```python
from build123d import *

# Parameters (mm, degrees)
BOSS_EXTRUDE1_DEPTH = 10
CUT_EXTRUDE5_REACH  = 103.397
SKETCH9_R           = 1.5
FILLET13_R          = 7.5
FILLET14_R          = 15
FILLET16_R          = 7.5
FILLET18_R          = 7.5
FILLET19_R          = 7.5
FILLET22_R          = 3
FILLET23_R          = 3
FILLET24_R          = 15
FILLET28_R          = 3
FILLET29_R          = 3
FILLET30_R          = 3
FILLET31_R          = 3
FILLET32_R          = 7.5
FILLET34_R          = 7.5
FILLET35_R          = 2.5
FILLET36_R          = 2.5


with BuildPart() as part:
    # Sketch1 → Boss-Extrude1 (new body)
    with BuildSketch(Plane(origin=(0, 0, 0), x_dir=(1, 0, 0), z_dir=(0, 1, 0))):
        with BuildLine():
            Line((0, -12.5), (0, -60))
            Line((0, -60), (22.5, -60))
            Line((22.5, -60), (81.125, -22.5))
            Line((81.125, -22.5), (81.125, 0))
            Line((81.125, 0), (75.125, 0))
            ThreePointArc((75.125, 0), (62.625, -12.5), (50.125, 0))
            Line((50.125, 0), (44.125, 0))
            Line((44.125, 0), (44.125, -12.5))
            Line((44.125, -12.5), (0, -12.5))
        make_face()
        Polygon((39.125, -17.5), (45.538841531, -34.595428821), (22.483333333, -50), (5, -50), (5, -17.5), align=None, mode=Mode.SUBTRACT)
        Polygon((71.125, -17.5), (49.69624181, -31.817655806), (44.125, -17.5), align=None, mode=Mode.SUBTRACT)
    boss_extrude1 = extrude(amount=BOSS_EXTRUDE1_DEPTH)

    # Mirror1: Boss-Extrude1 across plane
    add(boss_extrude1.mirror(Plane(origin=(0, 10, 0), x_dir=(0, 0, 1), z_dir=(-1, 0, 0))))

    # Sketch9 → Cut-Extrude5 (cut, up to next)
    with BuildSketch(Plane.XY.offset(60), mode=Mode.PRIVATE) as cut_extrude5_sk1:
        with Locations((-17.75, 5)):
            Circle(SKETCH9_R)
    cut_extrude5_tool1 = extrude(cut_extrude5_sk1.sketch, amount=-CUT_EXTRUDE5_REACH, mode=Mode.PRIVATE) & part.part
    cut_extrude5 = cut_extrude5_tool1.solids().sort_by_distance((-17.75, 5, 60))[0]
    add(cut_extrude5, mode=Mode.SUBTRACT)

    # Mirror2: Cut-Extrude5 across plane
    add(cut_extrude5.mirror(Plane(origin=(0, 0, 0), x_dir=(0, 0, 1), z_dir=(1, 0, 0))), mode=Mode.SUBTRACT)

    # Fillet13
    fillet13_edges = [part.edges().sort_by_distance(p)[0] for p in [
        (39.125, 5, 17.5),
    ]]
    fillet(fillet13_edges, radius=FILLET13_R)

    # Fillet14
    fillet14_edges = [part.edges().sort_by_distance(p)[0] for p in [
        (45.538841531, 5, 34.595428821),
    ]]
    fillet(fillet14_edges, radius=FILLET14_R)

    # Fillet16
    fillet16_edges = [part.edges().sort_by_distance(p)[0] for p in [
        (5, 5, 17.5),
    ]]
    fillet(fillet16_edges, radius=FILLET16_R)

    # Fillet18
    fillet18_edges = [part.edges().sort_by_distance(p)[0] for p in [
        (-5, 5, 17.5),
    ]]
    fillet(fillet18_edges, radius=FILLET18_R)

    # Fillet19
    fillet19_edges = [part.edges().sort_by_distance(p)[0] for p in [
        (-39.125, 5, 17.5),
    ]]
    fillet(fillet19_edges, radius=FILLET19_R)

    # Fillet22
    fillet22_edges = [part.edges().sort_by_distance(p)[0] for p in [
        (44.125, 5, 12.5),
    ]]
    fillet(fillet22_edges, radius=FILLET22_R)

    # Fillet23
    fillet23_edges = [part.edges().sort_by_distance(p)[0] for p in [
        (-44.125, 5, 12.5),
    ]]
    fillet(fillet23_edges, radius=FILLET23_R)

    # Fillet24
    fillet24_edges = [part.edges().sort_by_distance(p)[0] for p in [
        (-45.538841531, 5, 34.595428821),
    ]]
    fillet(fillet24_edges, radius=FILLET24_R)

    # Fillet28
    fillet28_edges = [part.edges().sort_by_distance(p)[0] for p in [
        (22.5, 5, 60),
    ]]
    fillet(fillet28_edges, radius=FILLET28_R)

    # Fillet29
    fillet29_edges = [part.edges().sort_by_distance(p)[0] for p in [
        (-22.5, 5, 60),
    ]]
    fillet(fillet29_edges, radius=FILLET29_R)

    # Fillet30
    fillet30_edges = [part.edges().sort_by_distance(p)[0] for p in [
        (81.125, 5, 22.5),
    ]]
    fillet(fillet30_edges, radius=FILLET30_R)

    # Fillet31
    fillet31_edges = [part.edges().sort_by_distance(p)[0] for p in [
        (-81.125, 5, 22.5),
    ]]
    fillet(fillet31_edges, radius=FILLET31_R)

    # Fillet32
    fillet32_edges = [part.edges().sort_by_distance(p)[0] for p in [
        (-5, 5, 50),
    ]]
    fillet(fillet32_edges, radius=FILLET32_R)

    # Fillet34
    fillet34_edges = [part.edges().sort_by_distance(p)[0] for p in [
        (5, 5, 50),
    ]]
    fillet(fillet34_edges, radius=FILLET34_R)

    # Fillet35
    fillet35_edges = [part.edges().sort_by_distance(p)[0] for p in [
        (-22.483333333, 5, 50),
    ]]
    fillet(fillet35_edges, radius=FILLET35_R)

    # Fillet36
    fillet36_edges = [part.edges().sort_by_distance(p)[0] for p in [
        (22.483333333, 5, 50),
    ]]
    fillet(fillet36_edges, radius=FILLET36_R)


solid = part.part
```
Could you check a few things on this model? Use its own coordinates, in mm. A direction names the side the tool comes from. Round coordinates to 2 decimals unless told otherwise and drop trailing zeros. Loops run counter-clockwise (first coordinate to the right, second up) from the corner with the lowest first, then second, coordinate; pieces in that order, holes last. Notation, with made-up numbers: M -7,86 L 18,86 A27 ccw 18,110 Z; hole C 44.5,-33.75 d11. An arc over 180 degrees is marked long. Answer as CSV lines item,"result".
1) We'd pull the mould along Z, two halves only. Please class faces 4 (the cylindrical face through (-62.9, 4.93, 12.497)), 5 (the flat face through (-51.09, 4.93, 41.71)), 6 (the cylindrical face through (41.64, 5.07, 33.19)): released by +Z, released by -Z, zero draft, split by the parting line, or undercut.
From the geometry:
face 4,"released by -Z"
face 5,"released by +Z"
face 6,"undercut"
2) Imagine slicing it at C-C on x = -48. List the corners of the cut face in (y, z) for me.
From the geometry:
outline,"M 0,0 L 10,0 L 10,17.5 L 0,17.5 Z; M 0,27.46 L 10,27.46 L 10,43.69 L 0,43.69 Z"
3) Imagine slicing it at A-A on x = 17.75. List the corners of the cut face in (y, z) for me, and give its area (3 significant figures).
From the geometry:
outline,"M 0,12.5 L 10,12.5 L 10,17.5 L 0,17.5 Z; M 0,50 L 3.5,50 L 3.5,60 L 0,60 Z; M 6.5,50 L 10,50 L 10,60 L 6.5,60 Z"
area,"120 mm^2"
4) Imagine slicing it at D-D on y = 2. Count the separate pieces of the cut face and the enclosed holes in it, and give its area (3 significant figures).
From the geometry:
separate pieces,"1"
enclosed holes,"4"
area,"3,500 mm^2"
5) Imagine slicing it at B-B on z = 36.5. List the corners of the cut face in (x, y) for me.
From the geometry:
outline,"M -59.24,0 L -40.15,0 L -40.15,10 L -59.24,10 Z; M -5,0 L 5,0 L 5,10 L -5,10 Z; M 40.15,0 L 59.24,0 L 59.24,10 L 40.15,10 Z"
6) Which directions (+Z, -Z, +X, -X, +Y, -Y) give clear straight access to the entire face, cutting with the end or side of a thin tool? Please do faces 1 (the flat face through (-78, 5, 0)), 2 (the flat face through (29.47, 4.93, 45.33)), 3 (the cylindrical face through (-43.223, 5.07, 11.645)).
From the geometry:
face 1,"-Z, +X, -X, +Y, -Y"
face 2,"+Y, -Y"
face 3,"-Z, +Y, -Y"
7) If I drill on probe 1 along Y at (x, z) = (17.75, 55.25); probe 2 along X at (y, z) = (7.5, 34); probe 3 along X at (y, z) = (9.5, 47.5) (3 decimals), over which ranges is the centre line in solid material (lowest first)?
From the geometry:
probe 1,"0 to 3.5, 6.5 to 10"
probe 2,"-63.15 to -41.36, -5 to 5, 41.36 to 63.15"
probe 3,"-42.042 to -26.225, -6.91 to 6.91, 26.225 to 42.042"
8) For pin 1 Ø2.5 at (x, y) = (17.75, 5) entering from +Z; pin 2 Ø3 at (y, z) = (3, 32) entering from -X; pin 3 Ø4 at (x, y) = (29.5, 2.5) entering from -Z; pin 4 Ø3 at (x, z) = (59, 38.5) entering from +Y, each with a flat end and sliding along its axis, tell me the tip position at first contact or that it passes through.
From the geometry:
pin 1,"z = 17.5"
pin 2,"x = -68.62"
pin 3,"z = 12.5"
pin 4,"through"
